Design review of the part built by this model. Coordinates are the model's own, in mm. A direction names the side the tool comes from. Coordinates: 2 decimals unless noted, no trailing zeros. Loops run counter-clockwise (first coordinate to the right, second up) from the corner with the lowest first, then second, coordinate; pieces in that order, holes last. Notation, with made-up numbers: (66.25, 73) -> (82.25, 73) arc R12 cw to (82.25, 95) -> close; hole circle Ø3 at (53.25, 68). An arc over 180 degrees is marked (long way). Answer in a Markdown table with one row per item.
```python
from build123d import *

# Parameters (mm, degrees)
BOSS_EXTRU_1_DEPTH                = 10.3
ESQUISSE3_W                       = 7
ESQUISSE3_H                       = 20.6
ESQUISSE3_R                       = 2.1
BOSS_EXTRU_2_DEPTH                = 3.2
BOSS_EXTRU_3_DEPTH                = 0.85
ESQUISSE8_R                       = 6.75
BOSS_EXTRU_7_DEPTH                = 1
ESQUISSE5_R                       = 2.925
BOSS_EXTRU_4_DEPTH                = 4.3
CONG_1_R                          = 2
ESQUISSE6_W                       = 3
ESQUISSE6_H                       = 6.8
BOSS_EXTRU_5_DEPTH                = 5.3
ESQUISSE7_R                       = 0.75
BOSS_EXTRU_6_DEPTH                = 5.3
DIAM_TRE_DU_PER_AGE_3_0_3_1_D     = 3
DIAM_TRE_DU_PER_AGE_3_0_3_1_DEPTH = 6
DIAM_TRE_DU_PER_AGE_3_0_3_1_TIP   = 0.901290929


with BuildPart() as part:
    # Esquisse1 → Boss.-Extru.1 (new, symmetric)
    with BuildSketch(Plane(origin=(0, 0, 0), x_dir=(1, 0, 0), z_dir=(0, 1, 0))):
        Polygon((-17.25, 9.3), (17.25, 9.3), (20.25, 6.3), (20.25, -28.2), (-20.25, -28.2), (-20.25, 6.3), align=None)
    extrude(amount=BOSS_EXTRU_1_DEPTH, both=True)

    # Esquisse3 → Boss.-Extru.2 (add)
    # profile 1 of 2: a face of its own
    with BuildSketch(Plane.XY.offset(3.5)):
        with Locations((23.75, 0)):
            Rectangle(ESQUISSE3_W, ESQUISSE3_H)
        with Locations((24.75, 5)):
            Circle(ESQUISSE3_R, mode=Mode.SUBTRACT)
        with Locations(Location((24.75, -5, 0), (0, 0, 180))):
            Circle(ESQUISSE3_R, mode=Mode.SUBTRACT)
    # profile 2 of 2: a face of its own
    with BuildSketch(Plane.XY.offset(3.5)):
        with Locations((-23.75, 0)):
            Rectangle(ESQUISSE3_W, ESQUISSE3_H)
        with Locations(Location((-24.75, 5, 0), (0, 0, 180))):
            Circle(ESQUISSE3_R, mode=Mode.SUBTRACT)
        with Locations((-24.75, -5)):
            Circle(ESQUISSE3_R, mode=Mode.SUBTRACT)
    extrude(amount=-BOSS_EXTRU_2_DEPTH)

    # Esquisse4 → Boss.-Extru.3 (add, symmetric)
    with BuildSketch(Plane(origin=(0, 0, 0), x_dir=(1, 0, 0), z_dir=(0, 1, 0))):
        Polygon((20.25, -0.3), (20.25, 1.6), (21.65, 1.6), (25.9, 0.2), (25.9, -0.3), align=None)
        Polygon((-25.9, -0.3), (-20.25, -0.3), (-20.25, 1.6), (-21.65, 1.6), (-25.9, 0.2), align=None)
    extrude(amount=BOSS_EXTRU_3_DEPTH, both=True)

    # Esquisse8 → Boss.-Extru.7 (add)
    with BuildSketch(Plane(origin=(0, 0, -9.3), x_dir=(-1, 0, 0), z_dir=(0, 0, -1))):
        with Locations(Location((10, 0, 0), (0, 0, 180))):
            Circle(ESQUISSE8_R)
    extrude(amount=BOSS_EXTRU_7_DEPTH)

    # Esquisse5 → Boss.-Extru.4 (add)
    with BuildSketch(Plane(origin=(0, 0, -10.3), x_dir=(-1, 0, 0), z_dir=(0, 0, -1))):
        with Locations(Location((10, 0, 0), (0, 0, 180))):
            Circle(ESQUISSE5_R)
    extrude(amount=BOSS_EXTRU_4_DEPTH)

    # Congé1
    cong_1_edges = [part.edges().sort_by_distance(p)[0] for p in [
        (27.25, 10.3, 1.9),
        (27.25, -10.3, 1.9),
        (-27.25, -10.3, 1.9),
        (-27.25, 10.3, 1.9),
    ]]
    fillet(cong_1_edges, radius=CONG_1_R)

    # Esquisse6 → Boss.-Extru.5 (add)
    with BuildSketch(Plane.ZY.offset(20.25)):
        with Locations((21.4, 0)):
            Rectangle(ESQUISSE6_W, ESQUISSE6_H)
    extrude(amount=BOSS_EXTRU_5_DEPTH)

    # Esquisse7 → Boss.-Extru.6 (add)
    with BuildSketch(Plane.ZY.offset(25.55)):
        with Locations((21.4, 0)):
            Circle(ESQUISSE7_R)
        with Locations((21.4, 1.6)):
            Circle(ESQUISSE7_R)
        with Locations(Location((21.4, -1.6, 0), (0, 0, 180))):
            Circle(ESQUISSE7_R)
    extrude(amount=BOSS_EXTRU_6_DEPTH)

    # Diamètre du perçage Ø3.0 (3)1
    with Locations(Plane(origin=(0, 0, -14.6), x_dir=(-1, 0, 0), z_dir=(0, 0, -1))):
        with Locations((10, 0)):
            Hole(DIAM_TRE_DU_PER_AGE_3_0_3_1_D / 2, depth=DIAM_TRE_DU_PER_AGE_3_0_3_1_DEPTH)
            with Locations((0, 0, -(DIAM_TRE_DU_PER_AGE_3_0_3_1_DEPTH + DIAM_TRE_DU_PER_AGE_3_0_3_1_TIP / 2))):  # 118° drill point
                Cone(0, DIAM_TRE_DU_PER_AGE_3_0_3_1_D / 2, DIAM_TRE_DU_PER_AGE_3_0_3_1_TIP, mode=Mode.SUBTRACT)


solid = part.part
```
(1) Take a section at A-A on x = -21. Give the boundary of the cut face in (y, z), and give its area (4 significant figures).
Evaluation:
| item | result |
|---|---|
| outline | (-10.3, 0.3) -> (-0.85, 0.3) -> (-0.85, -1.6) -> (0.85, -1.6) -> (0.85, 0.3) -> (10.3, 0.3) -> (10.3, 3.5) -> (-10.3, 3.5) -> close; (-3.4, 19.9) -> (3.4, 19.9) -> (3.4, 22.9) -> (-3.4, 22.9) -> close |
| area | 89.55 mm² |
(2) For pin 1 (1 mm diameter, centred on x = 17.5, y = 3.5, fed in from -Z); pin 2 (4 mm diameter, centred on y = 8, z = -4.5, fed in from -X); pin 3 (3.5 mm diameter, centred on y = -2.5, z = 2.5, fed in from -X), all flat-tipped, find the tip position at first contact; note any pin that passes through.
Evaluation:
| item | result |
|---|---|
| pin 1 | stops at z = -9.3 |
| pin 2 | stops at x = -20.25 |
| pin 3 | stops at x = -27.25 |
(3) To check wall thickness, follow probe 1 along Y at (x, z) = (24.75, 1.4); probe 2 along Z at (x, y) = (14.5, 5.25); probe 3 along Y at (x, z) = (24, 1). State the ranges of each line that lie inside material, in increasing order.
Evaluation:
| item | result |
|---|---|
| probe 1 | y = -10.3 to -7.1, -2.9 to 2.9, 7.1 to 10.3 |
| probe 2 | z = -9.3 to 28.2 |
| probe 3 | y = -10.3 to -6.96, -3.04 to 3.04, 6.96 to 10.3 |
(4) Tool access review of faces 5 (the flat face through (-25.55, 0.8, 22)), 6 (the flat face through (-23, 3.4, 21)), 7 (the cylindrical face through (-3.765, 2.585, -9.793)): name each direction out of +Z, -Z, +X, -X, +Y, -Y from which nothing blocks a thin tool from reaching the whole face with its end or side.
Evaluation:
| item | result |
|---|---|
| face 5 | -X |
| face 6 | +Z, -X, +Y |
| face 7 | -Z |
(5) Draft analysis for pull direction X (two halves, no side actions). For faces 1 (the cylindrical face through (-23.781, -6.863, 1.922)), 2 (the flat face through (-30.85, 0, 21)), 3 (the flat face through (18.73, 0.14, -7.82)), 4 (the cylindrical face through (-12.922, -0.129, -12.42)), state which applies: pulls with the +X half, pulls with the -X half, needs draft (parallel to the pull), parting line crosses it, or undercut.
Evaluation:
| item | result |
|---|---|
| face 1 | undercut |
| face 2 | pulls with the -X half |
| face 3 | pulls with the +X half |
| face 4 | parting line crosses it |
(6) Take a section at C-C on z = 21.4. Give the boundary of the cut face in (x, y), and give its area (3 significant figures).
Evaluation:
| item | result |
|---|---|
| outline | (-30.85, -2.35) -> (-25.55, -2.35) -> (-25.55, -3.4) -> (-20.25, -3.4) -> (-20.25, -10.3) -> (20.25, -10.3) -> (20.25, 10.3) -> (-20.25, 10.3) -> (-20.25, 3.4) -> (-25.55, 3.4) -> (-25.55, 2.35) -> (-30.85, 2.35) -> (-30.85, 0.85) -> (-25.55, 0.85) -> (-25.55, 0.75) -> (-30.85, 0.75) -> (-30.85, -0.75) -> (-25.55, -0.75) -> (-25.55, -0.85) -> (-30.85, -0.85) -> close |
| area | 894 mm² |
(7) Take a section at D-D on x = -14.5. Give the boundary of the cut face in (y, z), and give its area (3 significant figures).
Evaluation:
| item | result |
|---|---|
| outline | (-10.3, -9.3) -> (-5.03, -9.3) -> (-5.03, -10.3) -> (5.03, -10.3) -> (5.03, -9.3) -> (10.3, -9.3) -> (10.3, 28.2) -> (-10.3, 28.2) -> close |
| area | 783 mm² |
(8) Take a section at B-B on y = 5. Give the boundary of the cut face in (x, z), and give its area (3 significant figures).
Evaluation:
| item | result |
|---|---|
| outline | (-27.25, 0.3) -> (-26.85, 0.3) -> (-26.85, 3.5) -> (-27.25, 3.5) -> close; (-22.65, 0.3) -> (-20.25, 0.3) -> (-20.25, -6.3) -> (-17.25, -9.3) -> (-14.53, -9.3) -> (-14.53, -10.3) -> (-5.47, -10.3) -> (-5.47, -9.3) -> (17.25, -9.3) -> (20.25, -6.3) -> (20.25, 0.3) -> (22.65, 0.3) -> (22.65, 3.5) -> (20.25, 3.5) -> (20.25, 28.2) -> (-20.25, 28.2) -> (-20.25, 3.5) -> (-22.65, 3.5) -> close; (26.85, 0.3) -> (27.25, 0.3) -> (27.25, 3.5) -> (26.85, 3.5) -> close |
| area | 1,540 mm² |
